Geometry check sheet. Reference: the model listing, model coordinates, mm. Round coordinates to 2 decimals unless told otherwise and drop trailing zeros. Write each loop counter-clockwise with the first axis right and the second up, starting at its lowest first coordinate (ties: lowest second). Pieces come first, ordered by that corner, then holes. Notation, with made-up numbers: (21, -35.5) - (47, -35.5) arc R27 cw to (47, -0.5) - close; hole circle Ø1 at (-16, 28.25). An arc over 180 degrees is marked (long way). Return JSON: item names as keys, results as strings.
```python
from build123d import *

# Parameters (mm, degrees)
SKETCH1_W                = 15
SKETCH1_H                = 60
BOSS_EXTRUDE2_DEPTH      = 39.11
BOSS_EXTRUDE3_DEPTH      = 12
BOSS_EXTRUDE3_DEPTH_BACK = 27
SKETCH3_W                = 60
SKETCH3_H                = 5
RIB1_REACH               = 55.008
SKETCH5_WALL_W           = 127.334599132
SKETCH5_WALL_H           = 10
SKETCH6_R                = 1.5
CUT_EXTRUDE2_DEPTH       = 50.434219929
SKETCH7_W                = 16
SKETCH7_H                = 16
CUT_EXTRUDE3_DEPTH       = 57.201353187
SKETCH8_R                = 1.75
CUT_EXTRUDE4_DEPTH       = 75.228310637
FILLET1_R                = 3
CUT_EXTRUDE5_DEPTH       = 75.228310637
SKETCH11_W               = 15
SKETCH11_H               = 10.608893068
CUT_EXTRUDE6_DEPTH       = 67.293605272


with BuildPart() as part:
    # Sketch1 → Boss-Extrude2 (new body)
    with BuildSketch(Plane(origin=(0, 0, 0), x_dir=(1, 0, 0), z_dir=(0, 1, 0))):
        Rectangle(SKETCH1_W, SKETCH1_H)
    extrude(amount=BOSS_EXTRUDE2_DEPTH)

    # Sketch3 → Boss-Extrude3 (add, two sides: drawn at the far end of the back side and taken through both)
    with BuildSketch(Plane.ZY.offset(7.5).offset(-BOSS_EXTRUDE3_DEPTH_BACK)):
        with Locations((0, 2.5)):
            Rectangle(SKETCH3_W, SKETCH3_H)
    extrude(amount=BOSS_EXTRUDE3_DEPTH + BOSS_EXTRUDE3_DEPTH_BACK)

    # Sketch5 wall → Rib1 (add, up to next)
    with BuildSketch(Plane(origin=(-12.037058369, 13.5275, 0), x_dir=(-0.46970610176, -0.882822846311, 0), z_dir=(0.882822846311, -0.46970610176, 0)), mode=Mode.PRIVATE) as rib1_sk1:
        Rectangle(SKETCH5_WALL_W, SKETCH5_WALL_H)
    rib1_tool1 = extrude(rib1_sk1.sketch, amount=RIB1_REACH, mode=Mode.PRIVATE) - part.part
    rib1 = rib1_tool1.solids().sort_by_distance((-12.037058369, 13.5275, 0))[0]
    add(rib1)

    # Sketch6 → Cut-Extrude2 (cut, through all)
    with BuildSketch(Plane(origin=(0, 5, 0), x_dir=(1, 0, 0), z_dir=(0, 1, 0))):
        with Locations(Location((-14.5, -25, 0), (0, 0, 270))):
            Circle(SKETCH6_R)
        with Locations(Location((-14.5, 25, 0), (0, 0, 90))):
            Circle(SKETCH6_R)
    cut_extrude2 = extrude(amount=-CUT_EXTRUDE2_DEPTH, mode=Mode.SUBTRACT)

    # Mirror1: Rib1, Cut-Extrude2 across plane
    add(rib1.mirror(Plane(origin=(0, 0, 0), x_dir=(0, 0, 1), z_dir=(1, 0, 0))))
    add(cut_extrude2.mirror(Plane(origin=(0, 0, 0), x_dir=(0, 0, 1), z_dir=(1, 0, 0))), mode=Mode.SUBTRACT)

    # Sketch7 → Cut-Extrude3 (cut, through all)
    with BuildSketch(Plane.ZY.offset(7.5)):
        with Locations((15, 31.11)):
            Rectangle(SKETCH7_W, SKETCH7_H)
    cut_extrude3 = extrude(amount=-CUT_EXTRUDE3_DEPTH, mode=Mode.SUBTRACT)

    # Mirror2: Cut-Extrude3 across plane
    add(cut_extrude3.mirror(Plane.XY), mode=Mode.SUBTRACT)

    # Sketch8 → Cut-Extrude4 (cut, through all)
    with BuildSketch(Plane(origin=(0, 0, -30), x_dir=(-1, 0, 0), z_dir=(0, 0, -1))):
        with Locations(Location((0, 31.61, 0), (0, 0, 90))):
            Circle(SKETCH8_R)
    extrude(amount=-CUT_EXTRUDE4_DEPTH, mode=Mode.SUBTRACT)

    # Fillet1
    fillet1_edges = [part.edges().sort_by_distance(p)[0] for p in [
        (7.5, 5, 17.5),
        (-7.5, 5, -17.5),
        (-7.5, 5, 17.5),
        (-16.574116738, 5, 0),
        (7.5, 5, -17.5),
        (16.574116738, 5, 0),
    ]]
    fillet(fillet1_edges, radius=FILLET1_R)
    fillet1_2_edges = [part.edges().sort_by_distance(p)[0] for p in [
        (19.5, 2.5, -30),
        (19.5, 2.5, 30),
        (-19.5, 2.5, -30),
        (-19.5, 2.5, 30),
    ]]
    fillet(fillet1_2_edges, radius=FILLET1_R)

    # Sketch10 → Cut-Extrude5 (cut, through all)
    with BuildSketch(Plane.XY.offset(30)):
        Polygon((7.5, 28.501106932), (-7.5, 28.501106932), (-22.220470771, 28.501106932), (-22.220470771, 0), (19.5, 0), (19.5, 28.501106932), align=None)
    extrude(amount=-CUT_EXTRUDE5_DEPTH, mode=Mode.SUBTRACT)


with BuildPart() as cut_extrude5_piece_1:
    # of the separate pieces the step leaves, piece 1, a body of its own (cut_extrude5_pieces)
    add(part.part.solids().sort_by_distance((7.5, 39.11, 7))[0])


with BuildPart() as cut_extrude5_piece_2:
    # of the separate pieces the step leaves, piece 2, a body of its own (cut_extrude5_pieces)
    add(part.part.solids().sort_by_distance((7.5, 28.501106932, 30))[0])


with BuildPart() as cut_extrude5_piece_3:
    # of the separate pieces the step leaves, piece 3, a body of its own (cut_extrude5_pieces)
    add(part.part.solids().sort_by_distance((-7.5, 28.501106932, -30))[0])


with BuildPart() as cut_extrude6_tool:
    # Sketch11 → Cut-Extrude6 (new, through all)
    with BuildSketch(Plane(origin=(0, 0, 23), x_dir=(-1, 0, 0), z_dir=(0, 0, -1))):
        with Locations((0, 33.805553466)):
            Rectangle(SKETCH11_W, SKETCH11_H)
    extrude(amount=CUT_EXTRUDE6_DEPTH)


with BuildPart() as cut_extrude5_piece_1_1:
    add(cut_extrude5_piece_1.part)

    # Cut-Extrude6: cut by cut_extrude6_tool
    add(cut_extrude6_tool.part, mode=Mode.SUBTRACT)


with BuildPart() as cut_extrude5_piece_3_1:
    add(cut_extrude5_piece_3.part)

    # Cut-Extrude6: cut by cut_extrude6_tool
    add(cut_extrude6_tool.part, mode=Mode.SUBTRACT)


solid = cut_extrude5_piece_2.part
```
(1) Section check A-A, the plane x = 0. Enter the section's corners in (y, z).
Response values:
{"outline": "(28.5, 23) - (29.86, 23) - (29.86, 30) - (28.5, 30) - close; (33.36, 23) - (39.11, 23) - (39.11, 30) - (33.36, 30) - close"}
(2) Material ranges on line 1 along X through (y, z) = (31.61, 25.25); line 2 along X through (y, z) = (30, 26); line 3 along Y through (x, z) = (-0.5, 26.75), recorded low to high. Write a range as [from, to].
Response values:
{"line 1": "x = [-7.5, -1.75], [1.75, 7.5]", "line 2": "x = [-7.5, -0.69], [0.69, 7.5]", "line 3": "y = [28.5, 29.93], [33.29, 39.11]"}
(3) Section check C-C, the plane z = 26.75. Enter the section's corners in (x, y), plus the area to 3 significant figures.
Response values:
{"outline": "(-7.5, 28.5) - (7.5, 28.5) - (7.5, 39.11) - (-7.5, 39.11) - close; hole circle Ø3.5 at (0, 31.61)", "area": "150 mm^2"}
(4) Release check for a two-part mould opening along X. For faces 1 (the face through (-0.67, 33.227, 26.451)), 2 (the face through (7.5, 34, 27)), 3 (the face through (0, 39.11, 26)) record: pulls with the +X half, pulls with the -X half, needs draft (parallel to the pull), parting line crosses it, or undercut.
Response values:
{"face 1": "undercut", "face 2": "pulls with the +X half", "face 3": "needs draft"}
(5) Gauge pin test, flat end, axial feed: pin 1 (6 mm diameter, centred on x = -1, y = 31, fed in from -Z). Record the tip position at first contact, or that the pin passes through.
Response values:
{"pin 1": "stops at z = 23"}
(6) Section check B-B, the plane y = 31.61. Enter the section's corners in (x, z).
Response values:
{"outline": "(-7.5, 23) - (-1.75, 23) - (-1.75, 30) - (-7.5, 30) - close; (1.75, 23) - (7.5, 23) - (7.5, 30) - (1.75, 30) - close"}
